```python
from build123d import *

# Parameters (mm, degrees)
F1_DEPTH  = 25
F3_DEPTH  = 2
F5_DEPTH  = 2
F6_DEPTH  = 25
F7_W      = 50
F7_H      = 20
F8_DEPTH  = 20.001
F9_R      = 2.5
F10_DEPTH = 25.001
F12_DEPTH = 25
F14_R     = 8.25
F15_DEPTH = 20
F16_R     = 2.5
F17_DEPTH = 25
F18_R     = 2.5
F19_DEPTH = 25
F21_R     = 4
F22_DEPTH = 17.5
F23_R     = 2.5
F24_DEPTH = 12.5


with BuildPart() as f1:
    # F0 (on Front) → F1 (new body)
    with BuildSketch(Plane.XZ):
        with BuildLine():
            Line((200, 20), (0, 20))
            Line((0, 20), (0, 0))
            Line((0, 0), (168.732845779, -20.7177883789))
            ThreePointArc((168.732845779, -20.7177883789), (177.2579638449, -22.5298581628), (185.3389035957, -25.7947697515))
            Line((185.3389035957, -25.7947697515), (274.4395560146, -71.1938197255))
            Line((274.4395560146, -71.1938197255), (312.6376562235, -53.3503712549))
            Line((312.6376562235, -53.3503712549), (214.3394109088, 15.4788011072))
            ThreePointArc((214.3394109088, 15.4788011072), (207.5176449876, 18.8429237687), (200, 20))
        make_face()
    extrude(amount=-F1_DEPTH)

    # F2 (on face) → F3 (cut)
    with BuildSketch(Plane.XZ):
        with BuildLine():
            ThreePointArc((169.0984538092, -17.740149924), (178.1350789591, -19.6609438949), (186.700875095, -23.121750179))
            Line((186.700875095, -23.121750179), (274.4966924755, -67.8559534935))
            Line((274.4966924755, -67.8559534935), (306.6638017347, -52.829757076))
            Line((306.6638017347, -52.829757076), (212.6186815997, 13.0213449744))
            ThreePointArc((212.6186815997, 13.0213449744), (206.6155275891, 15.9817729165), (200, 17))
            Line((200, 17), (3, 17))
            Line((3, 17), (3, 2.6541757937))
            Line((3, 2.6541757937), (169.0984538092, -17.740149924))
        make_face()
    extrude(amount=-F3_DEPTH, mode=Mode.SUBTRACT)

    # F4 (on face) → F5 (cut)
    with BuildSketch(Plane(origin=(0, 25, 0), x_dir=(-1, 0, 0), z_dir=(0, 1, 0))):
        with BuildLine():
            ThreePointArc((-200, 17), (-206.6155275891, 15.9817729165), (-212.6186815997, 13.0213449744))
            Line((-212.6186815997, 13.0213449744), (-306.6638017347, -52.829757076))
            Line((-306.6638017347, -52.829757076), (-274.4966924755, -67.8559534935))
            Line((-274.4966924755, -67.8559534935), (-186.700875095, -23.121750179))
            ThreePointArc((-186.700875095, -23.121750179), (-178.1350789591, -19.6609438949), (-169.0984538092, -17.740149924))
            Line((-169.0984538092, -17.740149924), (-3, 2.6541757937))
            Line((-3, 2.6541757937), (-3, 17))
            Line((-3, 17), (-200, 17))
        make_face()
    extrude(amount=-F5_DEPTH, mode=Mode.SUBTRACT)

    # F0 (on Front) → F6 (join)
    with BuildSketch(Plane.XZ):
        with BuildLine():
            Line((0, 0), (0, 20))
            Line((0, 20), (-25.9173546986, 13.8933867464))
            ThreePointArc((-25.9173546986, 13.8933867464), (-29, 10), (-25.9173546986, 6.1066132536))
            Line((-25.9173546986, 6.1066132536), (0, 0))
        make_face()
    extrude(amount=-F6_DEPTH)

    # F7 (on Top) → F8 (cut, through all)
    with BuildSketch(Plane.XY):
        with Locations((-25, 12.5)):
            Rectangle(F7_W, F7_H)
    extrude(amount=F8_DEPTH, mode=Mode.SUBTRACT)

    # F9 (on Front) → F10 (cut, through all)
    with BuildSketch(Plane.XZ):
        with Locations((-19, 10)):
            Circle(F9_R)
    extrude(amount=-F10_DEPTH, mode=Mode.SUBTRACT)

    # F11 (on Front) → F12 (join)
    with BuildSketch(Plane.XZ):
        Polygon((150, 45), (150, 20), (200, 20), (193.1540331912, 44.0443909977), align=None)
    extrude(amount=-F12_DEPTH)

    # F14 (on face) → F15 (cut)
    with BuildSketch(Plane(origin=(150, 0, 0), x_dir=(0, -1, 0), z_dir=(-1, 0, 0))):
        with Locations((-12.5, 31.5)):
            Circle(F14_R)
    extrude(amount=-F15_DEPTH, mode=Mode.SUBTRACT)

    # F16 (on face) → F17 (cut)
    with BuildSketch(Plane.XZ):
        with Locations((144.0621566447, 31.638596327)):
            Circle(F16_R)
    extrude(amount=-F17_DEPTH, mode=Mode.SUBTRACT)

    # F18 (on face) → F19 (cut)
    with BuildSketch(Plane.XZ):
        with Locations((158, 31)):
            Circle(F18_R)
    extrude(amount=-F19_DEPTH, mode=Mode.SUBTRACT)

    # F21 (on offset) → F22 (join, symmetric)
    with BuildSketch(Plane.XZ.offset(-12.5)):
        with Locations((272.6376562235, -46.1938197255)):
            Circle(F21_R)
    extrude(amount=F22_DEPTH, both=True)

    # F23 (on offset) → F24 (cut, symmetric)
    with BuildSketch(Plane.XZ.offset(-12.5)):
        with Locations((140, 0)):
            Circle(F23_R)
    extrude(amount=F24_DEPTH, both=True, mode=Mode.SUBTRACT)


solid = f1.part
```
For this review, take the finished solid that the model builds, in its own axes (mm). A direction names the side the tool comes from. Give positions to 0.01 mm unless a question says otherwise; leave off trailing zeros. Loops run counter-clockwise (first coordinate to the right, second up) from the corner with the lowest first, then second, coordinate; pieces in that order, holes last. Notation, with made-up numbers: M 30,41 L 38,41 A8 cw 38,55 Z; hole C 5.5,-25 d7. An arc over 180 degrees is marked long. One line per item, written item: value. Start each with the question number.
Q1. Add section A-A (y = 12.5). Give the boundary of the cut face in (x, z), and give its area (3 significant figures).
Q2. Draft analysis for pull direction Z (two halves, no side actions). For faces 6 (the face through (229.984, 0.986, -45.176)), 7 (the face through (-11, 2.5, 10)), 8 (the face through (-12.78, 23.73, 16.99)), state which applies: released by +Z, released by -Z, zero draft, split by the parting line, or undercut.
Q3. Clearance check with flat-ended pins moving along their axes: pin 1 Ø4 at (x, z) = (-19, 10) entering from -Y; pin 2 Ø4 at (x, y) = (273.5, 3.5) entering from +Z; pin 3 Ø8 at (x, z) = (158, 31) entering from +Y; pin 4 Ø16 at (x, z) = (-17, 11) entering from -Y. State where each tip first meets the part, or that it passes through.
Q4. Add section C-C (z = -59.5). Give the boundary of the cut face in (x, y), and give its area (3 significant figures).
Q5. Machinability: for faces 1 (the face through (258.98, 24.01, -19.44)), 2 (the face through (-11, 22.5, 10)), 3 (the face through (150, 7, 38)), 4 (the face through (170, 13, 32)), 5 (the face through (290.355, 0.986, -60.448)), which of the approach directions +Z, -Z, +X, -X, +Y, -Y give a long, thin tool a straight path to every point of the face, cutting with its end or side? Answer none if there is none.
Q6. Add section B-B (x = 75). Give the boundary of the cut face in (y, z), and give its area (3 significant figures).
Q7. For L1, parallel to Y at x = 259.5, z = -46.5; L2, parallel to X at y = 23, z = 31; L3, parallel to Z at x = -19, y = 23.7, list the stretches that pass through material, from the lowest coordinate up.
Reply:
1. outline: M 0,0 L 168.73,-20.72 A50 cw 185.34,-25.79 L 274.44,-71.19 L 312.64,-53.35 L 214.34,15.48 A25 ccw 200,20 L 193.15,44.04 L 150,45 L 150,39.75 L 170,39.75 L 170,23.25 L 150,23.25 L 150,20 L 0,20 Z; hole C 140,0 d5
1. area: 12,000 mm²
2. face 6: undercut
2. face 7: zero draft
2. face 8: released by +Z
3. pin 1: through
3. pin 2: z = -24.55
3. pin 3: y = 25
3. pin 4: y = 0
4. outline: M 251.49,0 L 258.1,0 L 258.1,2 L 292.38,2 L 292.38,0 L 299.47,0 L 299.47,25 L 292.38,25 L 292.38,23 L 258.1,23 L 258.1,25 L 251.49,25 Z
4. area: 1,060 mm²
5. face 1: +Y
5. face 2: +Z, -Z, -X
5. face 3: +Z, -X, +Y, -Y
5. face 4: -X
5. face 5: -Y
6. outline: M 0,-9.21 L 25,-9.21 L 25,-6.19 L 23,-6.19 L 23,17 L 25,17 L 25,20 L 0,20 L 0,17 L 2,17 L 2,-6.19 L 0,-6.19 Z
6. area: 637 mm²
7. L1: 2 to 23
7. L2: 150 to 155.5, 160.5 to 196.87
7. L3: 4.48 to 7.5, 12.5 to 15.52
